```python
from build123d import *

# Parameters (mm, degrees)
F0_W         = 101
F0_H         = 80
F1_DEPTH     = 3
F2_R         = 25
F3_W         = 23
F3_H         = 69
F4_DEPTH     = 10
F5_R         = 10
F6_SIZE      = 5
F7_R         = 5
F8_T1_DEPTH  = 30
F8_T3_DEPTH  = 51
F8_T5_DEPTH  = 14
F8_T7_DEPTH  = 14
F8_T10_ANGLE = 90
F8_T12_ANGLE = 90
F8_T14_ANGLE = 90
F8_T16_ANGLE = 90


# Not quite as in the source:
# - a fillet or chamfer that OpenCascade refuses, or shapes differently, is made with other operations: its cross-section is extruded or revolved along the edge and cut away or added


with BuildPart() as f1:
    # F0 (on Top) → F1 (new body)
    with BuildSketch(Plane.XY):
        with Locations((0, 33.399283886)):
            Rectangle(F0_W, F0_H)
    extrude(amount=F1_DEPTH)

    # F2
    f2_edges = [f1.edges().sort_by_distance(p)[0] for p in [
        (50.5, -6.600716, 1.5),
        (50.5, 73.399284, 1.5),
        (-50.5, -6.600716, 1.5),
        (-50.5, 73.399284, 1.5),
    ]]
    fillet(f2_edges, radius=F2_R)

    # F3 (on Top) → F4 (join)
    with BuildSketch(Plane.XY):
        with Locations((0, -27.2368434817)):
            Rectangle(F3_W, F3_H)
    extrude(amount=F4_DEPTH)

    # F5
    f5_edges = [f1.edges().sort_by_distance(p)[0] for p in [
        (11.5, -61.736843, 5),
        (-11.5, -61.736843, 5),
    ]]
    fillet(f5_edges, radius=F5_R)

    # F6
    f6_edges = [f1.edges().sort_by_distance(p)[0] for p in [
        (0, 7.263157, 10),
    ]]
    chamfer(f6_edges, length=F6_SIZE)

    # F7
    f7_edges = [f1.edges().sort_by_distance(p)[0] for p in [
        (-11.5, -24.736843, 10),
    ]]
    fillet(f7_edges, radius=F7_R)

    # F8: chamfer of 5 on 1 edges, made by hand

    # F8_s2 → F8_t1 (cut)
    with BuildSketch(Plane.XZ.offset(-48.399283886)):
        Polygon((-45.5, 3), (-50.5, -2), (-50.5, 3), align=None)
        Polygon((45.5, 3), (50.5, -2), (50.5, 3), align=None)
    extrude(amount=F8_T1_DEPTH, mode=Mode.SUBTRACT)

    # F8_s4 → F8_t3 (cut)
    with BuildSketch(Plane.YZ.offset(-25.5)):
        Polygon((68.399283886, 3), (73.399283886, -2), (73.399283886, 3), align=None)
    extrude(amount=F8_T3_DEPTH, mode=Mode.SUBTRACT)

    # F8_s6 → F8_t5 (cut)
    with BuildSketch(Plane.YZ.offset(11.5)):
        Polygon((-1.600716114, 3), (-6.600716114, -2), (-6.600716114, 3), align=None)
    extrude(amount=F8_T5_DEPTH, mode=Mode.SUBTRACT)

    # F8_s8 → F8_t7 (cut)
    with BuildSketch(Plane.YZ.offset(-25.5)):
        Polygon((-6.600716114, -2), (-1.600716114, 3), (-6.600716114, 3), align=None)
    extrude(amount=F8_T7_DEPTH, mode=Mode.SUBTRACT)

    # F8_s9 → F8_t10 (revolve, cut)
    with BuildSketch(Plane.XZ.offset(-48.399283886)):
        Polygon((-45.5, 3), (-50.5, -2), (-50.5, 3), align=None)
    revolve(axis=Axis((-25.5, 48.399283886, 3), (0, 0, -1)), revolution_arc=F8_T10_ANGLE, mode=Mode.SUBTRACT)

    # F8_s11 → F8_t12 (revolve, cut)
    with BuildSketch(Plane.XZ.offset(-48.399283886)):
        Polygon((45.5, 3), (50.5, -2), (50.5, 3), align=None)
    revolve(axis=Axis((25.5, 48.399283886, 3), (0, 0, 1)), revolution_arc=F8_T12_ANGLE, mode=Mode.SUBTRACT)

    # F8_s13 → F8_t14 (revolve, cut)
    with BuildSketch(Plane.YZ.offset(25.5)):
        Polygon((-1.600716114, 3), (-6.600716114, -2), (-6.600716114, 3), align=None)
    revolve(axis=Axis((25.5, 18.399283886, 3), (0, 0, 1)), revolution_arc=F8_T14_ANGLE, mode=Mode.SUBTRACT)

    # F8_s15 → F8_t16 (revolve, cut)
    with BuildSketch(Plane.XZ.offset(-18.399283886)):
        Polygon((-45.5, 3), (-50.5, -2), (-50.5, 3), align=None)
    revolve(axis=Axis((-25.5, 18.399283886, 3), (0, 0, 1)), revolution_arc=F8_T16_ANGLE, mode=Mode.SUBTRACT)


solid = f1.part
```
Design review of the part built by this model. Coordinates are the model's own, in mm. A direction names the side the tool comes from. Round coordinates to 2 decimals unless told otherwise and drop trailing zeros. Order: outer loops, then holes, each group sorted by start corner. A loop starts at its lowest first (then second) coordinate and runs counter-clockwise, first axis right, second up. Notation, with made-up numbers: M -11.5,41 L 31.5,41 A32 cw 31.5,73 Z; hole C -25,13.25 d8. An arc over 180 degrees is marked long. Put each result on its own line as item: value.
Q1. To check wall thickness, follow line 1 (Z direction, x = -41.5, y = 52); line 2 (X direction, y = -46.5, z = 2.5); line 3 (X direction, y = -37.5, z = 9.5). State the ranges of each line that lie inside material, in increasing order.
Reported:
line 1: 0 to 3
line 2: -11.5 to 11.5
line 3: -8.68 to 8.68
Q2. Consider section A-A (y = -11). State the section outline as (x, z) points.
Reported:
outline: M -11.5,0 L 11.5,0 L 11.5,5 A5 ccw 6.5,10 L -6.5,10 A5 ccw -11.5,5 Z
Q3. Consider section B-B (x = -15). State the section outline as (y, z) points, and give its area (3 significant figures).
Reported:
outline: M -4.6,0 L 71.4,0 L 68.4,3 L -1.6,3 Z
area: 219 mm²
Q4. Machinability: for faces 1 (the face through (11.5, -22, 3)), 2 (the face through (-18.6, -3.1, 1.5)), 3 (the face through (8.49, -58.89, 2.54)), which of the approach directions +Z, -Z, +X, -X, +Y, -Y give a long, thin tool a straight path to every point of the face, cutting with its end or side? Answer none if there is none.
Reported:
face 1: +Z, +X, -Y
face 2: +Z, -X, -Y
face 3: +Z, -Z, +X, -Y
Q5. Consider section C-C (y = 28). State the section outline as (x, z) points.
Reported:
outline: M -48.5,0 L 48.5,0 L 45.5,3 L -45.5,3 Z
Q6. Insertion check: pin 1 Ø3 at (x, z) = (6, 6.5) entering from -Y; pin 2 Ø5.5 at (y, z) = (-15.5, 2.5) entering from -X; pin 3 Ø1.5 at (y, z) = (-36.5, 1.5) entering from +X. Each pin has a flat end and moves straight along its axis. Give the tip position at first contact, or say it passes through.
Reported:
pin 1: y = -61.15
pin 2: x = -11.5
pin 3: x = 11.5
